Geometry check sheet. Reference: the model listing, model coordinates, mm. A direction names the side the tool comes from. Give positions to 0.01 mm unless a question says otherwise; leave off trailing zeros. Loops run counter-clockwise (first coordinate to the right, second up) from the corner with the lowest first, then second, coordinate; pieces in that order, holes last. Notation, with made-up numbers: (69, 76) - (106, 76) arc R34 cw to (106, 106) - close; hole circle Ø11 at (6, 28.25). An arc over 180 degrees is marked (long way). Use a Markdown table: item, result. Add a question column.
1. Cross-section at D-D on y = 0. Count the separate pieces of the cut face and the enclosed holes in it, and give its area (3 significant figures).
2. Material ranges on L1, parallel to X at y = -1, z = 1.25; L2, parallel to Z at x = -9.5, y = 4.5; L3, parallel to Y at x = 4.5, z = 1.75, recorded low to high.
3. Cross-section at C-C on x = -9. Enter the section's corners in (y, z).
4. Set-up check for faces 4 (the flat face through (-4, 14, 1)), 5 (the flat face through (-8, 13, 14.65)), 6 (the flat face through (7, -1.65, 1)), 7 (the flat face through (5, 2, 2.5)): record each of +Z, -Z, +X, -X, +Y, -Y from which the full face is reachable in a straight line by a thin tool's end or side.
5. Cross-section at B-B on z = 13. Enter the section's corners in (x, y), and give its area (3 significant figures).
6. Depth check by flat-ended pin: P1, Ø3, axis at x = 5.5, z = 1, coming from the +Y side; P2, Ø10, axis at y = 9.5, z = 11, coming from the -X side; P3, Ø10.5, axis at x = -15.5, y = 11, coming from the +Z side. Enter the tip coordinate at first touch or a pass-through.
7. Draft check along Y on faces 1 (the flat face through (-8, 13, 11.35)), 2 (the cylindrical face through (-8.48, 19.14, 16.1)), 3 (the flat face through (-5, 5, 0)). Enter one of: pulls with the +Y half, pulls with the -Y half, needs draft (parallel to the pull), parting line crosses it, or undercut.
8. Cross-section at A-A on x = 15. Enter the section's corners in (y, z), and give its area (3 significant figures).
from build123d import *

# Parameters (mm, degrees)
SKETCH_1_W          = 42
SKETCH_1_H          = 40
EXTRUDE_1_DEPTH     = 2.5
SKETCH_2_W          = 3
SKETCH_2_H          = 25
EXTRUDE_2_DEPTH     = 14.5
CUT_EXTRUDE_2_DEPTH = 33.422985674
CUT_EXTRUDE_3_DEPTH = 39.379682125
SKETCH_6_W          = 42
SKETCH_6_H          = 15
CUT_EXTRUDE_4_DEPTH = 33.422985674
CUT_EXTRUDE_5_DEPTH = 33.422985674
FILLET_2_R          = 3
FILLET_3_SIZE       = 1.5
FILLET_4_R          = 1.5
FILLET_5_R          = 4


# Some blends are built 0.0001 mm under size
with BuildPart() as part:
    # 草图1 → 凸台-拉伸1 (new body)
    with BuildSketch(Plane.XY):
        Rectangle(SKETCH_1_W, SKETCH_1_H)
    extrude(amount=EXTRUDE_1_DEPTH)

    # 草图2 → 凸台-拉伸2 (add)
    with BuildSketch(Plane.XY.offset(2.5)):
        with Locations((-8.5, 7.5)):
            Rectangle(SKETCH_2_W, SKETCH_2_H)
    extrude(amount=EXTRUDE_2_DEPTH)

    # 草图5 → 切除-拉伸2 (cut, through all)
    with BuildSketch(Plane.XY.offset(2.5)):
        with BuildLine():
            Line((-18, 1.65), (-13.5, 1.65))
            ThreePointArc((-13.5, 1.65), (-11.85, 0), (-13.5, -1.65))
            Line((-13.5, -1.65), (-18, -1.65))
            ThreePointArc((-18, -1.65), (-19.65, 0), (-18, 1.65))
        make_face()
        with BuildLine():
            Line((-3.5, 1.65), (16.5, 1.65))
            ThreePointArc((16.5, 1.65), (18.15, 0), (16.5, -1.65))
            Line((16.5, -1.65), (-3.5, -1.65))
            ThreePointArc((-3.5, -1.65), (-5.15, 0), (-3.5, 1.65))
        make_face()
    extrude(amount=-CUT_EXTRUDE_2_DEPTH, mode=Mode.SUBTRACT)

    # 草图4 → 切除-拉伸3 (cut, through all)
    with BuildSketch(Plane(origin=(-7, 0, 0), x_dir=(0, 0, -1), z_dir=(1, 0, 0))):
        with BuildLine():
            Line((-11.35, 16), (-11.35, 10.5))
            ThreePointArc((-11.35, 10.5), (-13, 8.85), (-14.65, 10.5))
            Line((-14.65, 10.5), (-14.65, 16))
            ThreePointArc((-14.65, 16), (-13, 17.65), (-11.35, 16))
        make_face()
        with BuildLine():
            Line((-11.35, -1), (-11.35, 4.5))
            ThreePointArc((-11.35, 4.5), (-13, 6.15), (-14.65, 4.5))
            Line((-14.65, 4.5), (-14.65, -1))
            ThreePointArc((-14.65, -1), (-13, -2.65), (-11.35, -1))
        make_face()
    extrude(amount=-CUT_EXTRUDE_3_DEPTH, mode=Mode.SUBTRACT)

    # 草图6 → 切除-拉伸4 (cut, through all)
    with BuildSketch(Plane.XY.offset(2.5)):
        with Locations((0, -12.5)):
            Rectangle(SKETCH_6_W, SKETCH_6_H)
    extrude(amount=-CUT_EXTRUDE_4_DEPTH, mode=Mode.SUBTRACT)

    # 草图7 → 切除-拉伸5 (cut, through all)
    with BuildSketch(Plane.XY.offset(2.5)):
        with BuildLine():
            Line((-21, 20), (-13, 20))
            Line((-13, 20), (-13, 8.65))
            ThreePointArc((-13, 8.65), (-14.171572875, 5.821572875), (-17, 4.65))
            Line((-17, 4.65), (-21, 4.65))
            Line((-21, 4.65), (-21, 20))
        make_face()
        with BuildLine():
            Line((21, 20), (-4, 20))
            Line((-4, 20), (-4, 8.65))
            ThreePointArc((-4, 8.65), (-2.828427125, 5.821572875), (0, 4.65))
            Line((0, 4.65), (21, 4.65))
            Line((21, 4.65), (21, 20))
        make_face()
    extrude(amount=-CUT_EXTRUDE_5_DEPTH, mode=Mode.SUBTRACT)

    # 圆角2
    fillet_2_edges = [part.edges().sort_by_distance(p)[0] for p in [
        (-8.5, 20, 17),
        (-8.5, -5, 17),
    ]]
    fillet(fillet_2_edges, radius=FILLET_2_R)

    # 圆角3
    # a fillet whose section is not a circle: 1.5 mm, written as the material it adds along each edge
    with BuildSketch(Plane(origin=(-10, 20, 2.5), x_dir=(0, 0, 1), z_dir=(0, -1, 0)), Plane(origin=(-7, -5, 2.5), x_dir=(0, 0, 1), z_dir=(0, 1, 0))) as fillet_3_piece_1:
        with BuildLine():
            Bezier((FILLET_3_SIZE, 0), (0, 0), (0, FILLET_3_SIZE), weights=[1, 0.111111111, 1])
            Line((0, FILLET_3_SIZE), (0, 0))
            Line((0, 0), (FILLET_3_SIZE, 0))
        make_face()
    extrude(amount=25)

    # 圆角4
    fillet_4_edges = [part.edges().sort_by_distance(p)[0] for p in [
        (-4, 20, 1.25),
        (-13, 20, 1.25),
    ]]
    fillet(fillet_4_edges, radius=FILLET_4_R)

    # 圆角5
    fillet_5_edges = [part.edges().sort_by_distance(p)[0] for p in [
        (-21, -5, 1.25),
        (-21, 4.65, 1.25),
        (21, -5, 1.25),
        (21, 4.65, 1.25),
    ]]
    fillet(fillet_5_edges, radius=FILLET_5_R - 0.0001)  # a hair under: the kernel refuses the full size


solid = part.part
Values found:
| question | item | result |
|---|---|---|
| 1 | separate pieces | 4 |
| 1 | enclosed holes | 0 |
| 1 | area | 62.8 mm2 |
| 2 | L1 | x = -21 to -19.31, -12.19 to -4.81, 17.81 to 21 |
| 2 | L2 | z = 0 to 11.35, 14.65 to 17 |
| 2 | L3 | y = -5 to -1.65, 1.65 to 4.65 |
| 3 | outline | (-5, 0) - (20, 0) - (20, 14) arc R3 ccw to (17, 17) - (-2, 17) arc R3 ccw to (-5, 14) - close; hole (-1, 11.35) - (4.5, 11.35) arc R1.65 ccw to (4.5, 14.65) - (-1, 14.65) arc R1.65 ccw to start; hole (10.5, 11.35) - (16, 11.35) arc R1.65 ccw to (16, 14.65) - (10.5, 14.65) arc R1.65 ccw to start |
| 4 | face 4 | +Z, -Z, +X, +Y |
| 4 | face 5 | +X, -X |
| 4 | face 6 | +Z, -Z |
| 4 | face 7 | +Z, +X, +Y, -Y |
| 5 | outline | (-10, -5) - (-7, -5) - (-7, -2.65) - (-10, -2.65) - close; (-10, 6.15) - (-7, 6.15) - (-7, 8.85) - (-10, 8.85) - close; (-10, 17.65) - (-7, 17.65) - (-7, 20) - (-10, 20) - close |
| 5 | area | 22.2 mm2 |
| 6 | P1 | stops at y = 4.65 |
| 6 | P2 | stops at x = -10 |
| 6 | P3 | stops at z = 3.63 |
| 7 | face 1 | undercut |
| 7 | face 2 | pulls with the +Y half |
| 7 | face 3 | needs draft |
| 8 | outline | (-5, 0) - (-1.65, 0) - (-1.65, 2.5) - (-5, 2.5) - close; (1.65, 0) - (4.65, 0) - (4.65, 2.5) - (1.65, 2.5) - close |
| 8 | area | 15.9 mm2 |
